Source: CAD feature listing. Evaluate the final solid. Frame: model axes, mm. Coordinates: 2 decimals unless noted, no trailing zeros. Loops run counter-clockwise (first coordinate to the right, second up) from the corner with the lowest first, then second, coordinate; pieces in that order, holes last.
Item 1: Pull-direction query (Y, two-part tool) for faces 1 (the flat face through (0, -59.5, 0)), 2 (the cylindrical face through (-2.58, 37.54, 4.05)), 3 (the cylindrical face through (-2.58, -57.04, 4.05)), 4 (the cylindrical face through (5, -58, 0)); classes: +Y half, -Y half, draft (parallel to the pull), parting line (faces both ways), or undercut.
Item 2: Section query A-A, the plane y = -53. Return the cut outline in (x, z), then the cut area to 3 significant figures.
Item 3: Line query: probe 1 along Y at (x, z) = (-4.5, -2); probe 2 along Z at (x, y) = (3, -12); probe 3 along X at (y, z) = (20, 0.5). Output: solid intervals per line, ascending.
```python
from build123d import *

# Parameters (mm, degrees)
CHAMFER_1_SIZE      = 1
CUT_EXTRUDE_START   = -3
SKETCH_2_R          = 5
SKETCH_2_R_2        = 4.8
CUT_EXTRUDE_1_DEPTH = 1.1


with BuildPart() as part:
    # 草图1 → 旋转1 (revolve)
    with BuildSketch(Plane.XY, mode=Mode.PRIVATE) as revolve_1_sk:
        Polygon((0, 40), (5, 40), (5, 30), (5, -49.5), (5, -59.5), (0, -59.5), align=None)
    revolve(revolve_1_sk.sketch.rotate(Axis((0, 40, 0), (0, -1, 0)), 180), axis=Axis((0, 40, 0), (0, -1, 0)))

    # 倒角1
    chamfer_1_edges = [part.edges().sort_by_distance(p)[0] for p in [
        (5, -59.5, 0),
        (5, 40, 0),
    ]]
    chamfer(chamfer_1_edges, length=CHAMFER_1_SIZE)

    # 草图2 → 切除-拉伸1 (cut)
    with BuildSketch(Plane(origin=(0, 40, 0), x_dir=(1, 0, 0), z_dir=(0, 1, 0)).offset(CUT_EXTRUDE_START)):
        with Locations(Location((0, 0, 0), (0, 0, 180))):
            Circle(SKETCH_2_R)
        with Locations(Location((0, 0, 0), (0, 0, 180))):
            Circle(SKETCH_2_R_2, mode=Mode.SUBTRACT)
    cut_extrude_1 = extrude(amount=CUT_EXTRUDE_1_DEPTH, mode=Mode.SUBTRACT)

    # 镜向1: 切除-拉伸1 across plane
    add(cut_extrude_1.mirror(Plane.ZX.offset(-9.75)), mode=Mode.SUBTRACT)


solid = part.part
```
Verdict:
1. face 1: -Y half
1. face 2: undercut
1. face 3: undercut
1. face 4: draft
2. outline: circle Ø10 at (0, 0)
2. area: 78.5 mm2
3. probe 1: y = -58.58 to -57.6, -56.5 to 37, 38.1 to 39.08
3. probe 2: z = -4 to 4
3. probe 3: x = -4.97 to 4.97
